Verification items for this drawing (mm, ordinates from the low corner). Round coordinates to 2 decimals unless told otherwise and drop trailing zeros. Loops run counter-clockwise (first coordinate to the right, second up) from the corner with the lowest first, then second, coordinate; pieces in that order, holes last. Notation, with made-up numbers: M 77,34.5 L 107,34.5 A6 cw 107,41.5 Z; hole C 17.25,19.5 d8. An arc over 180 degrees is marked long. Use one line per item in the form item = value. Start each with the question number.
1. Cross-section at C-C (y = 5.75). State how many separate pieces and enclosed holes the cut face has, then the cut area to 3 significant figures.
2. Go/stop test with flat-tipped pins: pin 1 (9 mm diameter, centred on x = 144.78, z = 144.78, fed in from -Y); pin 2 (18 mm diameter, centred on x = 104.37, z = 185.19, fed in from +Y). Record where each tip stops, or that it passes through.
3. Cross-section at A-A (z = 144.78). Record the boundary of the cut face in (x, y) (1 decimal), then the cut area to 3 significant figures.
4. Material ranges on line 1 (Z direction, x = 41, y = 1.5) (1 decimal); line 2 (Z direction, x = 216.5, y = 8.5); line 3 (X direction, y = 5.25, z = 164.5), recorded low to high.
5. Cross-section at B-B (x = 144.78). Record the boundary of the cut face in (y, z) (1 decimal).
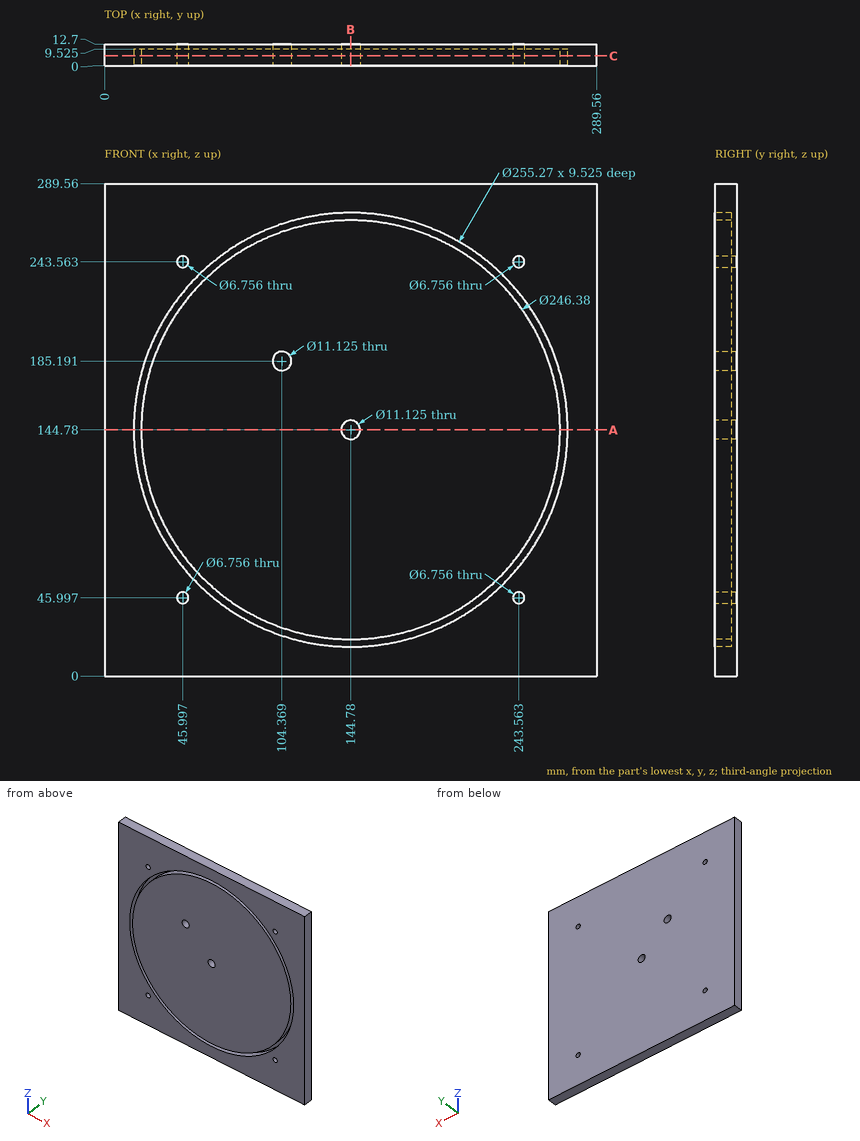
Reported:
q1.separate_pieces = 2
q1.enclosed_holes = 7
q1.area = 80,000 mm²
q2.pin_1 = through
q2.pin_2 = 12.7
q3.outline = M 0,0 L 17.1,0 L 17.1,9.5 L 21.6,9.5 L 21.6,0 L 139.2,0 L 139.2,12.7 L 0,12.7 Z; M 150.3,0 L 268,0 L 268,9.5 L 272.4,9.5 L 272.4,0 L 289.6,0 L 289.6,12.7 L 150.3,12.7 Z
q3.area = 3,450 mm²
q4.line_1 = 0 to 70.5, 78.4 to 211.2, 219.1 to 289.6
q4.line_2 = 0 to 39.2, 44.62 to 244.94, 250.36 to 289.56
q4.line_3 = 0 to 18.68, 23.18 to 266.38, 270.88 to 289.56
q5.outline = M 0,0 L 12.7,0 L 12.7,139.2 L 0,139.2 L 0,21.6 L 9.5,21.6 L 9.5,17.1 L 0,17.1 Z; M 0,150.3 L 12.7,150.3 L 12.7,289.6 L 0,289.6 L 0,272.4 L 9.5,272.4 L 9.5,268 L 0,268 Z
